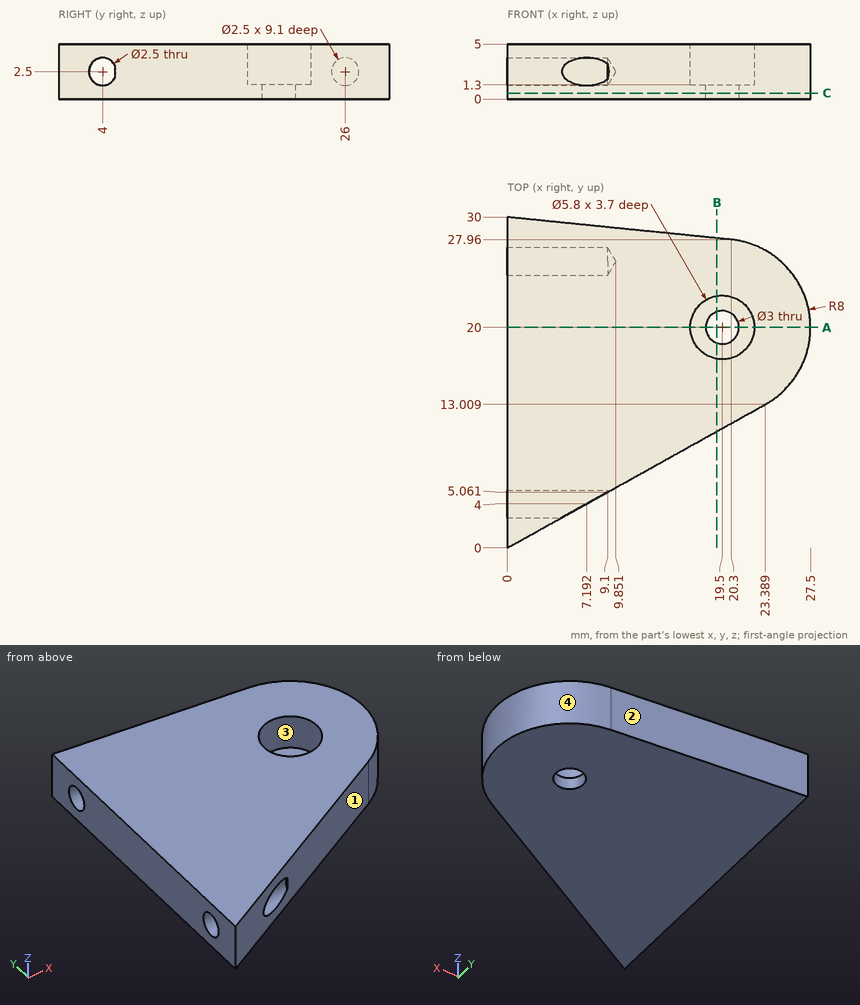
Can you work these out from the drawing? Everything is in mm from the part's minimum corner. Coordinates: 2 decimals unless noted, no trailing zeros. Loops run counter-clockwise (first coordinate to the right, second up) from the corner with the lowest first, then second, coordinate; pieces in that order, holes last. Notation, with made-up numbers: (10.5, 85) - (48.5, 85) arc R9 ccw to (48.5, 93) - close; hole circle Ø4 at (-16.75, -2). An arc over 180 degrees is marked (long way). Answer as CSV lines item,"result".
Q1. For pin 1 (3 mm diameter, centred on y = 4, z = 2.5, fed in from +X); pin 2 (2 mm diameter, centred on y = 26, z = 2.5, fed in from +X) (1 decimal); pin 3 (1 mm diameter, centred on x = 16.5, z = 4, fed in from -Y), each with a flat end and sliding along its axis, tell me the tip position at first contact or that it passes through.
Response:
pin 1,"x = 9.89"
pin 2,"x = 25.7"
pin 3,"y = 8.9"
Q2. If we section it at C-C, the plane z = 0.55: Write out the boundary of the cut face in (x, y).
Response:
outline,"(0, 0) - (23.39, 13.01) arc R8 ccw to (20.3, 27.96) - (0, 30) - close; hole circle Ø3 at (19.5, 20)"
Q3. If we section it at B-B, the plane x = 19: Write out the boundary of the cut face in (y, z) (1 decimal), and give its area (3 significant figures).
Response:
outline,"(10.6, 0) - (18.6, 0) - (18.6, 1.3) - (17.1, 1.3) - (17.1, 5) - (10.6, 5) - close; (21.4, 0) - (28.1, 0) - (28.1, 5) - (22.9, 5) - (22.9, 1.3) - (21.4, 1.3) - close"
area,"62.8 mm2"
Q4. If I drill on L1, parallel to Z at x = 6.5, y = 26; L2, parallel to X at y = 17.75, z = 4.7 (1 decimal); L3, parallel to Y at x = 5.25, z = 2.5, over which ranges is the centre line in solid material (lowest first)? Write a range as [from, to].
Response:
L1,"[0, 1.25], [3.75, 5]"
L2,"[0, 17.7], [21.3, 27.2]"
L3,"[5.25, 24.75], [27.25, 29.47]"
Q5. If we section it at A-A, the plane y = 20: Write out the boundary of the cut face in (x, z), and give its area (3 significant figures).
Response:
outline,"(0, 0) - (18, 0) - (18, 1.3) - (16.6, 1.3) - (16.6, 5) - (0, 5) - close; (21, 0) - (27.5, 0) - (27.5, 5) - (22.4, 5) - (22.4, 1.3) - (21, 1.3) - close"
area,"112 mm2"
Q6. We'd pull the mould along Y, two halves only. Please class the marked faces 1, 2, 3 and 4: pulls with the +Y half, pulls with the -Y half, needs draft (parallel to the pull), parting line crosses it, or undercut.
Response:
face 1,"pulls with the -Y half"
face 2,"pulls with the +Y half"
face 3,"undercut"
face 4,"parting line crosses it"
